```python
from build123d import *

# Parameters (mm, degrees)
CROQUIS1_W              = 1200
CROQUIS1_H              = 950
SALIENTE_EXTRUIR1_DEPTH = 20
CROQUIS2_W              = 150
CROQUIS2_H              = 180
CORTAR_EXTRUIR1_DEPTH   = 20
CROQUIS3_W              = 600
CROQUIS3_H              = 500
CORTAR_EXTRUIR2_DEPTH   = 20
CROQUIS5_W              = 1200
CROQUIS5_H              = 300
CORTAR_EXTRUIR4_DEPTH   = 40
CROQUIS4_R              = 11.5
CORTAR_EXTRUIR5_DEPTH   = 40
CROQUIS6_W              = 80
CROQUIS6_H              = 650
CROQUIS6_W_2            = 178
CORTAR_EXTRUIR6_DEPTH   = 30
CROQUIS7_W              = 2
CROQUIS7_H              = 650
CORTAR_EXTRUIR7_DEPTH   = 30


with BuildPart() as part:
    # Croquis1 → Saliente-Extruir1 (new body)
    with BuildSketch(Plane.XY):
        Rectangle(CROQUIS1_W, CROQUIS1_H)
    extrude(amount=SALIENTE_EXTRUIR1_DEPTH)

    # Croquis2 → Cortar-Extruir1 (cut)
    with BuildSketch(Plane.XY.offset(20)):
        with Locations((-200, 355)):
            Rectangle(CROQUIS2_W, CROQUIS2_H)
    extrude(amount=-CORTAR_EXTRUIR1_DEPTH, mode=Mode.SUBTRACT)

    # Croquis3 → Cortar-Extruir2 (cut)
    with BuildSketch(Plane(origin=(0, 0, 0), x_dir=(-1, 0, 0), z_dir=(0, 0, -1))):
        with Locations((-120, -165)):
            Rectangle(CROQUIS3_W, CROQUIS3_H)
    extrude(amount=-CORTAR_EXTRUIR2_DEPTH, mode=Mode.SUBTRACT)

    # Croquis5 → Cortar-Extruir4 (cut)
    with BuildSketch(Plane(origin=(0, 0, 0), x_dir=(-1, 0, 0), z_dir=(0, 0, -1))):
        with Locations((0, 325)):
            Rectangle(CROQUIS5_W, CROQUIS5_H)
    extrude(amount=-CORTAR_EXTRUIR4_DEPTH, mode=Mode.SUBTRACT)

    # Croquis4 → Cortar-Extruir5 (cut)
    with BuildSketch(Plane(origin=(0, 0, 0), x_dir=(-1, 0, 0), z_dir=(0, 0, -1))):
        with Locations((-50, 145)):
            Circle(CROQUIS4_R)
    extrude(amount=-CORTAR_EXTRUIR5_DEPTH, mode=Mode.SUBTRACT)

    # Croquis6 → Cortar-Extruir6 (cut)
    with BuildSketch(Plane(origin=(0, 0, 0), x_dir=(-1, 0, 0), z_dir=(0, 0, -1))):
        with Locations((-560, -150)):
            Rectangle(CROQUIS6_W, CROQUIS6_H)
        with Locations((511, -150)):
            Rectangle(CROQUIS6_W_2, CROQUIS6_H)
    extrude(amount=-CORTAR_EXTRUIR6_DEPTH, mode=Mode.SUBTRACT)

    # Croquis7 → Cortar-Extruir7 (cut)
    with BuildSketch(Plane(origin=(0, 0, 0), x_dir=(-1, 0, 0), z_dir=(0, 0, -1))):
        with Locations((421, -150)):
            Rectangle(CROQUIS7_W, CROQUIS7_H)
    extrude(amount=-CORTAR_EXTRUIR7_DEPTH, mode=Mode.SUBTRACT)


solid = part.part
```
Here's how the part is built. I have some questions about the finished solid (model axes, mm). A direction names the side the tool comes from. Coordinates: 2 decimals unless noted, no trailing zeros. Write each loop counter-clockwise with the first axis right and the second up, starting at its lowest first coordinate (ties: lowest second). Pieces come first, ordered by that corner, then holes. Notation, with made-up numbers: M -10,-27.75 L 23,-27.75 A13 ccw 23,-22.75 Z; hole C -39,13.5 d7. An arc over 180 degrees is marked long. Answer as CSV lines item,"result". Start each with the question number.
Q1. Suppose I cut it at C-C, the plane x = 243. List the corners of the cut face in (y, z) for me, then the cut area to 3 significant figures.
Q2. For faces 4 (the flat face through (124, -415, 10)), 5 (the flat face through (-270, -145, 20)), which set-ups out of +Z, -Z, +X, -X, +Y, -Y let a thin tool reach every point of the face, with its end or its side?
Q3. Suppose I cut it at D-D, the plane z = 4.75. List the corners of the cut face in (x, y) for me.
Q4. I need wall thicknesses on probe 1 along Y at (x, z) = (50, 7.75); probe 2 along X at (y, z) = (-65.5, 12.5); probe 3 along Y at (x, z) = (113.5, 16.75). Which ranges of each line are inside material? Lowest first, please. Write a range as [from, to].
Q5. If we mould it in two halves opening along Y, with no side actions, what happens to faces 1 (the cylindrical face through (58.48, 152.77, 9.86)), 2 (the flat face through (520, -155, 10)), 3 (the flat face through (43, -475, 10))? For each: pulls with the +Y half, pulls with the -Y half, needs draft (parallel to the pull), parting line crosses it, or undercut.
Q6. Suppose I cut it at B-B, the plane y = 145. List the corners of the cut face in (x, z) for me, then the cut area to 3 significant figures.
Q7. Suppose I cut it at A-A, the plane x = 50. List the corners of the cut face in (y, z) for me.
Entries:
1,outline,"M -475,0 L -415,0 L -415,20 L -475,20 Z; M 85,0 L 175,0 L 175,20 L 85,20 Z"
1,area,"3,000 mm²"
2,face 4,"+Z, -Z"
2,face 5,"+Z, +X, -X, +Y, -Y"
3,outline,"M -420,-475 L 520,-475 L 520,175 L -420,175 Z; hole M -180,-415 L 420,-415 L 420,85 L -180,85 Z; hole C 50,145 d23"
4,probe 1,"y = [-475, -415], [85, 133.5], [156.5, 175]"
4,probe 2,"x = [-420, -180], [420, 520]"
4,probe 3,"y = [-475, -415], [85, 175]"
5,face 1,"undercut"
5,face 2,"needs draft"
5,face 3,"pulls with the -Y half"
6,outline,"M -420,0 L 38.5,0 L 38.5,20 L -420,20 Z; M 61.5,0 L 520,0 L 520,20 L 61.5,20 Z"
6,area,"18,300 mm²"
7,outline,"M -475,0 L -415,0 L -415,20 L -475,20 Z; M 85,0 L 133.5,0 L 133.5,20 L 85,20 Z; M 156.5,0 L 175,0 L 175,20 L 156.5,20 Z"
